Here's how the part is built. I have some questions about the finished solid (model axes, mm). Face numbers are marked on the shaded views. A direction names the side the tool comes from. Give positions to 0.01 mm unless a question says otherwise; leave off trailing zeros. Write each loop counter-clockwise with the first axis right and the second up, starting at its lowest first coordinate (ties: lowest second). Pieces come first, ordered by that corner, then holes. Notation, with made-up numbers: (9.5, 83) -> (65.5, 83) arc R6 ccw to (65.5, 92) -> close; hole circle Ø6 at (33, 6.25). An arc over 180 degrees is marked (long way). Return JSON: item names as keys, results as strings.
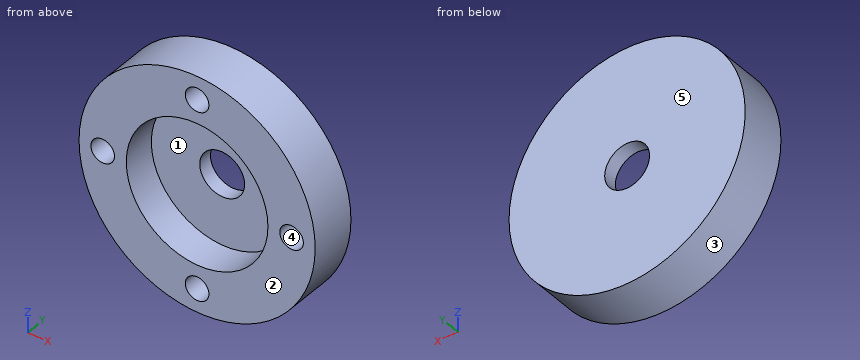
from build123d import *

# Parameters (mm, degrees)
F0_R     = 25
F1_DEPTH = 10
F2_R     = 4.75
F3_DEPTH = 25
F4_R     = 15
F5_DEPTH = 7
F7_D     = 5
F7_DEPTH = 6
F7_TIP   = 1.5021515476


with BuildPart() as f1:
    # F0 (on Front) → F1 (new body)
    with BuildSketch(Plane.XZ):
        Circle(F0_R)
    extrude(amount=F1_DEPTH)

    # F2 (on face) → F3 (cut)
    with BuildSketch(Plane.XZ.offset(10)):
        Circle(F2_R)
    extrude(amount=-F3_DEPTH, mode=Mode.SUBTRACT)

    # F4 (on face) → F5 (cut)
    with BuildSketch(Plane.XZ.offset(10)):
        Circle(F4_R)
    extrude(amount=-F5_DEPTH, mode=Mode.SUBTRACT)

    # F7
    with Locations(Plane.XZ.offset(10)):
        with Locations((0, 20), (20, 0), (0, -20), (-20, 0)):
            Hole(F7_D / 2, depth=F7_DEPTH)
            with Locations((0, 0, -(F7_DEPTH + F7_TIP / 2))):  # 118° drill point
                Cone(0, F7_D / 2, F7_TIP, mode=Mode.SUBTRACT)


solid = f1.part
1. Suppose I cut it at B-B, the plane z = 6. List the corners of the cut face in (x, y) for me, and give its area (3 significant figures).
Taken from the geometry:
{"outline": "(-24.27, -10) -> (-13.75, -10) -> (-13.75, -3) -> (13.75, -3) -> (13.75, -10) -> (24.27, -10) -> (24.27, 0) -> (-24.27, 0) -> close", "area": "293 mm²"}
2. For pin 1 Ø4 at (x, y) = (12, -1.5) entering from +Z; pin 2 Ø2 at (x, y) = (-12, -6.5) entering from +Z; pin 3 Ø1 at (x, z) = (8.5, -0.5) entering from -Y, each with a flat end and sliding along its axis, tell me the tip position at first contact or that it passes through.
Taken from the geometry:
{"pin 1": "stops at z = 22.91", "pin 2": "stops at z = 22.45", "pin 3": "stops at y = -3"}
3. If we mould it in two halves opening along Z, with no side actions, what happens to the marked faces 1, 2 and 3? For each: released by +Z, released by -Z, zero draft, split by the parting line, or undercut.
Taken from the geometry:
{"face 1": "undercut", "face 2": "zero draft", "face 3": "split by the parting line"}
4. Suppose I cut it at A-A, the plane y = -9. List the corners of the cut face in (x, z) for me, and give its area (3 significant figures).
Taken from the geometry:
{"outline": "circle Ø50 at (0, 0); hole circle Ø5 at (-20, 0); hole circle Ø30 at (0, 0); hole circle Ø5 at (0, -20); hole circle Ø5 at (0, 20); hole circle Ø5 at (20, 0)", "area": "1,180 mm²"}
5. If I drill on line 1 (Z direction, x = 0, y = -7.7); line 2 (Z direction, x = -20, y = -5.5); line 3 (Z direction, x = -1.5, y = -3.75), over which ranges is the centre line in solid material (lowest first)? Write a range as [from, to].
Taken from the geometry:
{"line 1": "z = [-25, -22.5], [-17.5, -15], [15, 17.5], [22.5, 25]", "line 2": "z = [-15, -2.5], [2.5, 15]", "line 3": "z = [-24.95, -21.45], [-18.55, -14.92], [14.92, 18.55], [21.45, 24.95]"}
6. Suppose I cut it at C-C, the plane y = -1.75. List the corners of the cut face in (x, z) for me, and give its area (3 significant figures).
Taken from the geometry:
{"outline": "circle Ø50 at (0, 0); hole circle Ø9.5 at (0, 0)", "area": "1,890 mm²"}
7. Suppose I cut it at D-D, the plane x = -14. List the corners of the cut face in (y, z) for me.
Taken from the geometry:
{"outline": "(-10, -20.71) -> (0, -20.71) -> (0, 20.71) -> (-10, 20.71) -> (-10, 5.39) -> (-3, 5.39) -> (-3, -5.39) -> (-10, -5.39) -> close"}
8. Which directions (+Z, -Z, +X, -X, +Y, -Y) give clear straight access to the entire face, cutting with the end or side of a thin tool? Please do the marked faces 4 and 5.
Taken from the geometry:
{"face 4": "-Y", "face 5": "+Z, -Z, +X, -X, +Y"}
